CAD build for the part. Positions are in the model's coordinates, mm. A direction names the side the tool comes from. Round coordinates to 2 decimals unless told otherwise and drop trailing zeros. Loops run counter-clockwise (first coordinate to the right, second up) from the corner with the lowest first, then second, coordinate; pieces in that order, holes last.
```python
from build123d import *

# Parameters (mm, degrees)
SKETCH_1_R      = 5
EXTRUDE_1_DEPTH = 8
FILLET_1_R      = 3
FILLET_2_R      = 3
FILLET_3_R      = 3


with BuildPart() as part:
    # 草圖1 → 填料-伸長1 (new body)
    with BuildSketch(Plane.XY):
        with BuildLine():
            Line((58.954715367, 9.945218954), (10.953934927, 4.900133633))
            ThreePointArc((10.953934927, 4.900133633), (0, 12), (-10.953934927, 4.900133633))
            Line((-10.953934927, 4.900133633), (-58.954715367, 9.945218954))
            ThreePointArc((-58.954715367, 9.945218954), (-70, 0), (-58.954715367, -9.945218954))
            Line((-58.954715367, -9.945218954), (-10.953934927, -4.900133633))
            ThreePointArc((-10.953934927, -4.900133633), (0, -12), (10.953934927, -4.900133633))
            Line((10.953934927, -4.900133633), (58.954715367, -9.945218954))
            ThreePointArc((58.954715367, -9.945218954), (70, 0), (58.954715367, 9.945218954))
        make_face()
        Circle(SKETCH_1_R, mode=Mode.SUBTRACT)
    extrude(amount=EXTRUDE_1_DEPTH)

    # 圓角1
    fillet_1_edges = [part.edges().sort_by_distance(p)[0] for p in [
        (10.953934927, -4.900133633, 4),
        (-10.953934927, -4.900133633, 4),
        (-10.953934927, 4.900133633, 4),
        (10.953934927, 4.900133633, 4),
    ]]
    fillet(fillet_1_edges, radius=FILLET_1_R)

    # 圓角2
    fillet_2_edges = [part.edges().sort_by_distance(p)[0] for p in [
        (-70, 0, 8),
        (-35.948953134, -7.527215907, 8),
        (-35.948953134, 7.527215907, 8),
        (0, 12, 8),
        (0, -12, 8),
        (35.948953134, -7.527215907, 8),
        (-11.32982846, 5.388970193, 8),
        (-11.32982846, -5.388970193, 8),
        (11.32982846, -5.388970193, 8),
        (11.32982846, 5.388970193, 8),
        (70, 0, 8),
        (35.948953134, 7.527215907, 8),
    ]]
    fillet(fillet_2_edges, radius=FILLET_2_R)

    # 圓角3
    fillet_3_edges = [part.edges().sort_by_distance(p)[0] for p in [
        (35.948953134, 7.527215907, 0),
        (70, 0, 0),
        (-35.948953134, 7.527215907, 0),
        (0, 12, 0),
        (0, -12, 0),
        (35.948953134, -7.527215907, 0),
        (-11.32982846, 5.388970193, 0),
        (-11.32982846, -5.388970193, 0),
        (11.32982846, -5.388970193, 0),
        (11.32982846, 5.388970193, 0),
        (-35.948953134, -7.527215907, 0),
        (-70, 0, 0),
    ]]
    fillet(fillet_3_edges, radius=FILLET_3_R)


solid = part.part
```
Item 1: Cut at B-B, the plane x = 0. Give the cut face in (y, z).
Answers follow:
outline: (-12, 3) arc R3 ccw to (-9, 0) - (-5, 0) - (-5, 8) - (-9, 8) arc R3 ccw to (-12, 5) - close; (5, 0) - (9, 0) arc R3 ccw to (12, 3) - (12, 5) arc R3 ccw to (9, 8) - (5, 8) - close
Item 2: Probe line 1 (X direction, y = 0.5, z = 3.25); line 2 (Y direction, x = 0, z = 4.5); line 3 (Y direction, x = 0, z = 6.5). List the from-to ranges inside material, lowest first.
Answers follow:
line 1: x = -69.99 to -4.97, 4.97 to 69.99
line 2: y = -12 to -5, 5 to 12
line 3: y = -11.6 to -5, 5 to 11.6
Item 3: Cut at C-C, the plane z = 6.75. Give the cut face in (x, y) (3 decimals), plus the area to 3 significant figures.
Answers follow:
outline: (-59.014, -9.385) - (-13.002, -4.549) arc R3.563 cw to (-9.629, -6.17) arc R11.437 ccw to (9.629, -6.17) arc R3.563 cw to (13.002, -4.549) - (59.014, -9.385) arc R9.437 ccw (long way) to (59.014, 9.385) - (13.002, 4.549) arc R3.563 cw to (9.629, 6.17) arc R11.437 ccw to (-9.629, 6.17) arc R3.563 cw to (-13.002, 4.549) - (-59.014, 9.385) arc R9.437 ccw (long way) to start; hole circle Ø10 at (0, 0)
area: 1,970 mm2
Item 4: Two-plate mould, pull along X, no slides. Class faces 4 (the flat face through (36.27, 7.56, 3.99)), 5 (the flat face through (-1, -6, 0)), 6 (the cylindrical face through (-35.72, -6.64, 0.9)): released by +X, released by -X, zero draft, split by the parting line, or undercut.
Answers follow:
face 4: undercut
face 5: zero draft
face 6: undercut
Item 5: Cut at A-A, the plane y = 0. Give the cut face in (x, z), plus the area to 3 significant figures.
Answers follow:
outline: (-70, 3) arc R3 ccw to (-67, 0) - (-5, 0) - (-5, 8) - (-67, 8) arc R3 ccw to (-70, 5) - close; (5, 0) - (67, 0) arc R3 ccw to (70, 3) - (70, 5) arc R3 ccw to (67, 8) - (5, 8) - close
area: 1,030 mm2
Item 6: 3-axis set-ups, long thin cutter, end or side, ignore diameter. For faces 1 (the cylindrical face through (-35.72, -6.6, 7.14)), 2 (the cylindrical face through (-36.36, 6.71, 0.9)), 3 (the flat face through (-36.27, -7.56, 3.99)): which of +Z, -Z, +X, -X, +Y, -Y reach the whole face in a straight line?
Answers follow:
face 1: +Z, -Y
face 2: -Z, +Y
face 3: +Z, -Z, -Y
Item 7: Flat gauge pins, fed straight in: P1, Ø4, axis at x = 37.5, z = 4, coming from the -Y side; P2, Ø1.5, axis at y = -6, z = 3.5, coming from the -X side; P3, Ø4, axis at x = 32.5, z = 4, coming from the -Y side. Where does each tip first touch, or does it go through?
Answers follow:
P1: stops at y = -7.9
P2: stops at x = -68.51
P3: stops at y = -7.37
